from build123d import *

# Parameters (mm, degrees)
BOSS_EXTRU_1_DEPTH      = 12
ESQUISSE6_R             = 2.5
BOSS_EXTRU_2_DEPTH      = 9.5
BOSS_EXTRU_3_DEPTH      = 5
CONG_1_R                = 4
ESQUISSE8_R             = 2.5
ENL_V_MAT_EXTRU_1_DEPTH = 125.49859437
BOSS_EXTRU_4_DEPTH      = 19


with BuildPart() as part:
    # Esquisse1 → Boss.-Extru.1 (new body)
    with BuildSketch(Plane.XZ.offset(-8.7)):
        Polygon((38.5, 59), (41.5, 59), (41.5, 48.4), (0, 48.4), (0, 113.4), (41.5, 113.4), (41.5, 101.8), (38.5, 101.8), (16.5, 101.8), (16.5, 59), align=None)
        with BuildLine():
            Line((21.5, 57.7), (23.5, 57.7))
            ThreePointArc((23.5, 57.7), (25.8, 55.4), (23.5, 53.1))
            Line((23.5, 53.1), (21.5, 53.1))
            ThreePointArc((21.5, 53.1), (19.2, 55.4), (21.5, 57.7))
        make_face(mode=Mode.SUBTRACT)
        with BuildLine():
            Line((31.5, 57.7), (33.5, 57.7))
            ThreePointArc((33.5, 57.7), (35.8, 55.4), (33.5, 53.1))
            Line((33.5, 53.1), (31.5, 53.1))
            ThreePointArc((31.5, 53.1), (29.2, 55.4), (31.5, 57.7))
        make_face(mode=Mode.SUBTRACT)
        with BuildLine():
            Line((21.5, 107.7), (23.5, 107.7))
            ThreePointArc((23.5, 107.7), (25.8, 105.4), (23.5, 103.1))
            Line((23.5, 103.1), (21.5, 103.1))
            ThreePointArc((21.5, 103.1), (19.2, 105.4), (21.5, 107.7))
        make_face(mode=Mode.SUBTRACT)
        with BuildLine():
            Line((31.5, 107.7), (33.5, 107.7))
            ThreePointArc((33.5, 107.7), (35.8, 105.4), (33.5, 103.1))
            Line((33.5, 103.1), (31.5, 103.1))
            ThreePointArc((31.5, 103.1), (29.2, 105.4), (31.5, 107.7))
        make_face(mode=Mode.SUBTRACT)
    boss_extru_1 = extrude(amount=BOSS_EXTRU_1_DEPTH)

    # Symétrie1: Boss.-Extru.1 across plane
    add(boss_extru_1.mirror(Plane(origin=(0, 0, 0), x_dir=(0, 0, 1), z_dir=(1, 0, 0))))



with BuildPart() as body_2:
    # Esquisse6 → Boss.-Extru.2 (new, symmetric)
    with BuildSketch(Plane(origin=(0, 29.5, 0), x_dir=(1, 0, 0), z_dir=(0, 1, 0))):
        with BuildLine():
            Line((-7.424824728, -33.32967845), (7.424824728, -33.32967845))
            ThreePointArc((7.424824728, -33.32967845), (15.424824728, -41.32967845), (7.424824728, -49.32967845))
            Line((7.424824728, -49.32967845), (-7.424824728, -49.32967845))
            ThreePointArc((-7.424824728, -49.32967845), (-15.424824728, -41.32967845), (-7.424824728, -33.32967845))
        make_face()
        with Locations(Location((7.424824728, -41.32967845, 0), (0, 0, 270))):
            Circle(ESQUISSE6_R, mode=Mode.SUBTRACT)
        with Locations(Location((-7.424824728, -41.32967845, 0), (0, 0, 90))):
            Circle(ESQUISSE6_R, mode=Mode.SUBTRACT)
    extrude(amount=BOSS_EXTRU_2_DEPTH, both=True)


with BuildPart() as part_1:
    add(part.part)

    add(body_2.part)  # Boss.-Extru.3 merges body 2
    # Esquisse7 → Boss.-Extru.3 (add, symmetric)
    with BuildSketch(Plane(origin=(0, 0, 0), x_dir=(0, 0, -1), z_dir=(1, 0, 0))):
        Polygon((-49.32967845, 20), (-49.32967845, 39), (-64.32967845, 39), (-78.4, 8.7), (-48.4, 8.7), align=None)
    extrude(amount=BOSS_EXTRU_3_DEPTH, both=True)

    # Congé1
    cong_1_edges = [part_1.edges().sort_by_distance(p)[0] for p in [
        (41.5, 2.7, 48.4),
        (41.5, 2.7, 113.4),
        (-41.5, 2.7, 48.4),
        (-41.5, 2.7, 113.4),
    ]]
    fillet(cong_1_edges, radius=CONG_1_R)

    # Esquisse8 → Enlèv. mat.-Extru.1 (cut, through all)
    with BuildSketch(Plane(origin=(0, 8.7, 0), x_dir=(1, 0, 0), z_dir=(0, 1, 0))):
        with Locations(Location((-10, -88.9, 0), (0, 0, 180))):
            Circle(ESQUISSE8_R)
        with Locations(Location((-10, -100.9, 0), (0, 0, 180))):
            Circle(ESQUISSE8_R)
        with Locations(Location((10, -100.9, 0), (0, 0, 180))):
            Circle(ESQUISSE8_R)
        with Locations(Location((10, -88.9, 0), (0, 0, 180))):
            Circle(ESQUISSE8_R)
    extrude(amount=-ENL_V_MAT_EXTRU_1_DEPTH, mode=Mode.SUBTRACT)

    # Esquisse9 → Boss.-Extru.4 (add)
    with BuildSketch(Plane(origin=(0, 39, 0), x_dir=(1, 0, 0), z_dir=(0, 1, 0))):
        Polygon((-7.424824728, -49.32967845), (-5, -51.32967845), (-5, -49.32967845), align=None)
        Polygon((5, -51.32967845), (5, -49.32967845), (7.424824728, -49.32967845), align=None)
    extrude(amount=-BOSS_EXTRU_4_DEPTH)


solid = part_1.part
Geometry check sheet. Reference: the model listing, model coordinates, mm. A direction names the side the tool comes from. Round coordinates to 2 decimals unless told otherwise and drop trailing zeros. Loops run counter-clockwise (first coordinate to the right, second up) from the corner with the lowest first, then second, coordinate; pieces in that order, holes last.
Item 1: Mould release check, pull along X, two halves, no side actions. Record for faces 4 (the flat face through (41.5, 3, 56)), 5 (the flat face through (1, 3, 113.4)), 6 (the flat face through (-33, 3, 103.1)): pulls with the +X half, pulls with the -X half, needs draft (parallel to the pull), parting line crosses it, or undercut.
Item 2: Gauge pin test, flat ends, axial feed: pin 1 (12 mm diameter, centred on x = -27, z = 82.5, fed in from +Y); pin 2 (8 mm diameter, centred on x = 22.5, z = 99.5, fed in from -Y); pin 3 (5 mm diameter, centred on x = 25.5, y = 11, fed in from -Z); pin 4 (6.5 mm diameter, centred on x = -7.42, z = 41.33, fed in from -Y). Record the tip position at first contact, or that the pin passes through.
Item 3: Access from +Z, -Z, +X, -X, +Y, -Y to the whole of each face (thin tool, end or side, straight path). Record for faces 1 (the flat face through (-16.5, 3, 81)), 2 (the cylindrical face through (19.2, 2.78, 55.35)), 3 (the flat face through (-1, 3, 48.4)).
Item 4: Thickness scan on line 1 (Z direction, x = -22, y = 6.5); line 2 (Z direction, x = -21, y = -1) (3 decimals); line 3 (X direction, y = 0, z = 100). Record the ranges inside material, lowest first.
Item 5: Cross-section at A-A on x = 22.5. Record the boundary of the cut face in (y, z), then the cut area to 3 significant figures.
Item 6: Cross-section at B-B on z = 88.9. Record the boundary of the cut face in (x, y), then the cut area to 3 significant figures.
Item 7: Cross-section at D-D on z = 75. Record the boundary of the cut face in (x, y), then the cut area to 3 significant figures.
Item 8: Cross-section at C-C on y = 28. Record the boundary of the cut face in (x, z).
Answer sheet:
1. face 4: pulls with the +X half
1. face 5: needs draft
1. face 6: undercut
2. pin 1: passes through
2. pin 2: stops at y = -3.3
2. pin 3: stops at z = 48.4
2. pin 4: stops at y = 20
3. face 1: -X, +Y, -Y
3. face 2: +Y, -Y
3. face 3: -Z, +X, -X, -Y
4. line 1: z = 48.4 to 53.1, 57.7 to 59, 101.8 to 103.1, 107.7 to 113.4
4. line 2: z = 48.4 to 53.155, 57.645 to 59, 101.8 to 103.155, 107.645 to 113.4
4. line 3: x = -16.5 to -12.33, -7.67 to 7.67, 12.33 to 16.5
5. outline: (-3.3, 48.4) - (8.7, 48.4) - (8.7, 53.1) - (-3.3, 53.1) - close; (-3.3, 57.7) - (8.7, 57.7) - (8.7, 59) - (-3.3, 59) - close; (-3.3, 101.8) - (8.7, 101.8) - (8.7, 103.1) - (-3.3, 103.1) - close; (-3.3, 107.7) - (8.7, 107.7) - (8.7, 113.4) - (-3.3, 113.4) - close
5. area: 156 mm2
6. outline: (-16.5, -3.3) - (-12.5, -3.3) - (-12.5, 8.7) - (-16.5, 8.7) - close; (-7.5, -3.3) - (7.5, -3.3) - (7.5, 8.7) - (-7.5, 8.7) - close; (12.5, -3.3) - (16.5, -3.3) - (16.5, 8.7) - (12.5, 8.7) - close
6. area: 276 mm2
7. outline: (-16.5, -3.3) - (16.5, -3.3) - (16.5, 8.7) - (5, 8.7) - (5, 16.02) - (-5, 16.02) - (-5, 8.7) - (-16.5, 8.7) - close
7. area: 469 mm2
8. outline: (-7.42, 33.33) - (7.42, 33.33) arc R8 ccw to (7.42, 49.33) - (5, 51.33) - (5, 69.44) - (-5, 69.44) - (-5, 51.33) - (-7.42, 49.33) arc R8 ccw to start; hole circle Ø5 at (-7.42, 41.33); hole circle Ø5 at (7.42, 41.33)
